For this review, take the finished solid that the model builds, in its own axes (mm). Coordinates: 2 decimals unless noted, no trailing zeros. Write each loop counter-clockwise with the first axis right and the second up, starting at its lowest first coordinate (ties: lowest second). Pieces come first, ordered by that corner, then holes. Notation, with made-up numbers: (36, 23.5) - (78, 23.5) arc R33 ccw to (78, 62.5) - close; hole circle Ø7 at (4.5, 57). An arc over 180 degrees is marked (long way). Use one line per item in the form item = value. Start each with the question number.
1) We need section A-A (x = -55). Give the boundary of the cut face in (y, z).
2) We need section C-C (x = -145). Give the boundary of the cut face in (y, z).
3) For L1, parallel to Y at x = -15, z = 0.6; L2, parallel to X at y = 55, z = 0.85; L3, parallel to Y at x = -145, z = 1, list the stretches that pass through material, from the lowest coordinate up. Write a range as from..to.
4) We need section B-B (y = 15). Give the boundary of the cut face in (x, z), plus the area to 3 significant figures.
5) Insertion check: P1, Ø0.8, axis at y = 19.5, z = 1.5, coming from the -X side; P2, Ø5.5, axis at x = -15, y = 10, coming from the +Z side. Each pin has a flat end and moves straight along its axis. Give the tip position at first contact, or say it passes through.
6) We need section D-D (y = 23). Give the boundary of the cut face in (x, z), plus the area to 3 significant figures.
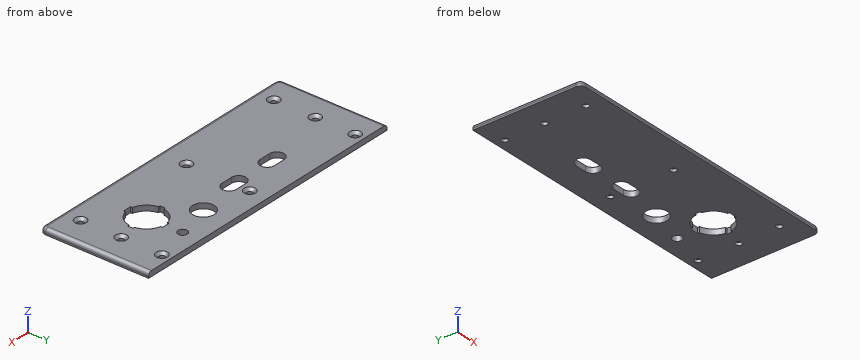
```python
from build123d import *

# Parameters (mm, degrees)
SKETCH11_W                                     = 160
SKETCH11_H                                     = 60
SKETCH11_R                                     = 2.55
SKETCH11_R_2                                   = 6
BOSS_EXTRUDE1_DEPTH                            = 3
FILLET1_R                                      = 2
FILLET3_R                                      = 3
CSK_FOR_M3_FLAT_HEAD_MACHINE_SCREW1_AT_2_COUNT = 2
CSK_FOR_M3_FLAT_HEAD_MACHINE_SCREW1_AT_2_PITCH = 22.022525482
CSK_FOR_M3_FLAT_HEAD_MACHINE_SCREW1_AT_3_COUNT = 2
CSK_FOR_M3_FLAT_HEAD_MACHINE_SCREW1_AT_3_PITCH = 45
CSK_FOR_M3_FLAT_HEAD_MACHINE_SCREW1_AT_4_COUNT = 2
CSK_FOR_M3_FLAT_HEAD_MACHINE_SCREW1_AT_4_PITCH = 137.490256535
CSK_FOR_M3_FLAT_HEAD_MACHINE_SCREW1_AT_5_COUNT = 2
CSK_FOR_M3_FLAT_HEAD_MACHINE_SCREW1_AT_5_PITCH = 131.892243209
CSK_FOR_M3_FLAT_HEAD_MACHINE_SCREW1_AT_6_COUNT = 2
CSK_FOR_M3_FLAT_HEAD_MACHINE_SCREW1_AT_6_PITCH = 130.000219213
CSK_FOR_M3_FLAT_HEAD_MACHINE_SCREW1_AT_7_COUNT = 2
CSK_FOR_M3_FLAT_HEAD_MACHINE_SCREW1_AT_7_PITCH = 65.174148425
CSK_FOR_M3_FLAT_HEAD_MACHINE_SCREW1_AT_8_COUNT = 2
CSK_FOR_M3_FLAT_HEAD_MACHINE_SCREW1_AT_8_PITCH = 76.196837301


with BuildPart() as part:
    # Sketch11 → Boss-Extrude1 (new body)
    with BuildSketch(Plane.XY):
        with Locations((-80, 30)):
            Rectangle(SKETCH11_W, SKETCH11_H)
        with Locations((-35, 50)):
            Circle(SKETCH11_R, mode=Mode.SUBTRACT)
        with Locations((-55, 45)):
            Circle(SKETCH11_R_2, mode=Mode.SUBTRACT)
        with BuildLine():
            Line((-44.886859967, 31.5), (-45.897247359, 31.5))
            Line((-45.897247359, 31.5), (-45.897247359, 28.5))
            Line((-45.897247359, 28.5), (-44.886859967, 28.5))
            ThreePointArc((-44.886859967, 28.5), (-42.370691635, 23.241826814), (-37.35, 20.280046296))
            Line((-37.35, 20.280046296), (-37.35, 19.253954216))
            Line((-37.35, 19.253954216), (-32.65, 19.253954216))
            Line((-32.65, 19.253954216), (-32.65, 20.280046296))
            ThreePointArc((-32.65, 20.280046296), (-27.629308365, 23.241826814), (-25.113140033, 28.5))
            Line((-25.113140033, 28.5), (-24.102752641, 28.5))
            Line((-24.102752641, 28.5), (-24.102752641, 31.5))
            Line((-24.102752641, 31.5), (-25.113140033, 31.5))
            ThreePointArc((-25.113140033, 31.5), (-27.629308365, 36.758173186), (-32.65, 39.719953704))
            Line((-32.65, 39.719953704), (-32.65, 40.746045784))
            Line((-32.65, 40.746045784), (-37.35, 40.746045784))
            Line((-37.35, 40.746045784), (-37.35, 39.719953704))
            ThreePointArc((-37.35, 39.719953704), (-42.370691635, 36.758173186), (-44.886859967, 31.5))
        make_face(mode=Mode.SUBTRACT)
        with BuildLine():
            Line((-83.627304882, 44.930328357), (-77.227304882, 44.930328357))
            ThreePointArc((-77.227304882, 44.930328357), (-73.227304882, 40.930328357), (-77.227304882, 36.930328357))
            Line((-77.227304882, 36.930328357), (-83.627304882, 36.930328357))
            ThreePointArc((-83.627304882, 36.930328357), (-87.627304882, 40.930328357), (-83.627304882, 44.930328357))
        make_face(mode=Mode.SUBTRACT)
        with BuildLine():
            Line((-109.252753418, 44.9), (-102.852753418, 44.9))
            ThreePointArc((-102.852753418, 44.9), (-98.852753418, 40.9), (-102.852753418, 36.9))
            Line((-102.852753418, 36.9), (-109.252753418, 36.9))
            ThreePointArc((-109.252753418, 36.9), (-113.252753418, 40.9), (-109.252753418, 44.9))
        make_face(mode=Mode.SUBTRACT)
    extrude(amount=BOSS_EXTRUDE1_DEPTH)

    # Fillet1
    fillet1_edges = [part.edges().sort_by_distance(p)[0] for p in [
        (-160, 30, 3),
        (-80, 0, 3),
        (0, 30, 3),
    ]]
    fillet(fillet1_edges, radius=FILLET1_R)

    # Fillet3
    # the kernel refuses this fillet: 3 mm, written as the material it takes off along each edge
    with BuildSketch(Plane(origin=(-3, 3, 3), x_dir=(0, -1, 0), z_dir=(-1, 0, 0))) as fillet3_piece_1:
        with BuildLine():
            CenterArc((1, -2), 2, 0, 90)
            Line((3, -2), (3, 0))
            Line((3, 0), (1, 0))
        make_face()
    revolve(axis=Axis((-3, 3, 3), (0, 0, 1)), revolution_arc=90, mode=Mode.SUBTRACT)
    with BuildSketch(Plane(origin=(-157, 3, 3), x_dir=(-1, 0, 0), z_dir=(0, 1, 0))) as fillet3_piece_2:
        with BuildLine():
            CenterArc((1, -2), 2, 0, 90)
            Line((3, -2), (3, 0))
            Line((3, 0), (1, 0))
        make_face()
    revolve(axis=Axis((-157, 3, 3), (0, 0, 1)), revolution_arc=90, mode=Mode.SUBTRACT)
    with BuildSketch(Plane(origin=(0, 0, -7.5), x_dir=(-1, 0, 0), z_dir=(0, 0, 1))) as fillet3_piece_3:
        with BuildLine():
            CenterArc((FILLET3_R, -FILLET3_R), FILLET3_R, 90, 90)
            Line((0, -FILLET3_R), (0, 0))
            Line((0, 0), (FILLET3_R, 0))
        make_face()
    extrude(amount=10.5, mode=Mode.SUBTRACT)
    with BuildSketch(Plane(origin=(-160, 0, -7.5), x_dir=(1, 0, 0), z_dir=(0, 0, 1))) as fillet3_piece_4:
        with BuildLine():
            CenterArc((FILLET3_R, FILLET3_R), FILLET3_R, 180, 90)
            Line((0, FILLET3_R), (0, 0))
            Line((0, 0), (FILLET3_R, 0))
        make_face()
    extrude(amount=10.5, mode=Mode.SUBTRACT)

    # Sketch13 → CSK for M3 Flat Head Machine Screw1 (revolve, cut)
    with BuildSketch(Plane(origin=(-145, 54.761262741, 3), x_dir=(0, -1, 0), z_dir=(1, 0, 0))):
        Polygon((0, 0), (0, 3), (1.7, 3), (1.7, 1.45), (3.15, 0), align=None)
    csk_for_m3_flat_head_machine_screw1 = revolve(axis=Axis((-145, 54.761262741, 9.35), (0, 0, -1)), mode=Mode.SUBTRACT)

    # CSK for M3 Flat Head Machine Screw1 at 2: CSK for M3 Flat Head Machine Screw1 ×2
    with Locations(*[(0, -i * CSK_FOR_M3_FLAT_HEAD_MACHINE_SCREW1_AT_2_PITCH, 0) for i in range(1, CSK_FOR_M3_FLAT_HEAD_MACHINE_SCREW1_AT_2_COUNT)]):
        add(csk_for_m3_flat_head_machine_screw1, mode=Mode.SUBTRACT)

    # CSK for M3 Flat Head Machine Screw1 at 3: CSK for M3 Flat Head Machine Screw1 ×2
    with Locations(*[(0, -i * CSK_FOR_M3_FLAT_HEAD_MACHINE_SCREW1_AT_3_PITCH, 0) for i in range(1, CSK_FOR_M3_FLAT_HEAD_MACHINE_SCREW1_AT_3_COUNT)]):
        add(csk_for_m3_flat_head_machine_screw1, mode=Mode.SUBTRACT)

    # CSK for M3 Flat Head Machine Screw1 at 4: CSK for M3 Flat Head Machine Screw1 ×2
    with Locations(*[Vector(0.9455215465875816, -0.3255595259528246, 0) * (i * CSK_FOR_M3_FLAT_HEAD_MACHINE_SCREW1_AT_4_PITCH) for i in range(1, CSK_FOR_M3_FLAT_HEAD_MACHINE_SCREW1_AT_4_COUNT)]):
        add(csk_for_m3_flat_head_machine_screw1, mode=Mode.SUBTRACT)

    # CSK for M3 Flat Head Machine Screw1 at 5: CSK for M3 Flat Head Machine Screw1 ×2
    with Locations(*[Vector(0.9856531122424032, -0.16878371463759412, 0) * (i * CSK_FOR_M3_FLAT_HEAD_MACHINE_SCREW1_AT_5_PITCH) for i in range(1, CSK_FOR_M3_FLAT_HEAD_MACHINE_SCREW1_AT_5_COUNT)]):
        add(csk_for_m3_flat_head_machine_screw1, mode=Mode.SUBTRACT)

    # CSK for M3 Flat Head Machine Screw1 at 6: CSK for M3 Flat Head Machine Screw1 ×2
    with Locations(*[Vector(0.9999983137474917, 0.0018364373589019598, 0) * (i * CSK_FOR_M3_FLAT_HEAD_MACHINE_SCREW1_AT_6_PITCH) for i in range(1, CSK_FOR_M3_FLAT_HEAD_MACHINE_SCREW1_AT_6_COUNT)]):
        add(csk_for_m3_flat_head_machine_screw1, mode=Mode.SUBTRACT)

    # CSK for M3 Flat Head Machine Screw1 at 7: CSK for M3 Flat Head Machine Screw1 ×2
    with Locations(*[Vector(0.9973279524332378, -0.0730544680038502, 0) * (i * CSK_FOR_M3_FLAT_HEAD_MACHINE_SCREW1_AT_7_PITCH) for i in range(1, CSK_FOR_M3_FLAT_HEAD_MACHINE_SCREW1_AT_7_COUNT)]):
        add(csk_for_m3_flat_head_machine_screw1, mode=Mode.SUBTRACT)

    # CSK for M3 Flat Head Machine Screw1 at 8: CSK for M3 Flat Head Machine Screw1 ×2
    with Locations(*[Vector(0.8530537788971958, -0.5218230066882967, 0) * (i * CSK_FOR_M3_FLAT_HEAD_MACHINE_SCREW1_AT_8_PITCH) for i in range(1, CSK_FOR_M3_FLAT_HEAD_MACHINE_SCREW1_AT_8_COUNT)]):
        add(csk_for_m3_flat_head_machine_screw1, mode=Mode.SUBTRACT)


solid = part.part
```
Determined:
q1.outline = (0, 0) - (39, 0) - (39, 3) - (2, 3) arc R2 ccw to (0, 1) - close; (51, 0) - (60, 0) - (60, 3) - (51, 3) - close
q2.outline = (0, 0) - (8.06, 0) - (8.06, 1.55) - (6.61, 3) - (2, 3) arc R2 ccw to (0, 1) - close; (11.46, 0) - (31.04, 0) - (31.04, 1.55) - (29.59, 3) - (12.91, 3) - (11.46, 1.55) - close; (34.44, 0) - (53.06, 0) - (53.06, 1.55) - (51.61, 3) - (35.89, 3) - (34.44, 1.55) - close; (56.46, 0) - (60, 0) - (60, 3) - (57.91, 3) - (56.46, 1.55) - close
q3.L1 = 0..8.3, 11.7..30.8, 34.2..53.3, 56.7..60
q3.L2 = -160..-146.68, -143.32..-16.7, -13.3..0
q3.L3 = 0..8.06, 11.46..31.04, 34.44..53.06, 56.46..60
q4.outline = (-160, 0) - (-81.7, 0) - (-81.7, 1.55) - (-83.15, 3) - (-158, 3) arc R2 ccw to (-160, 1) - close; (-78.3, 0) - (0, 0) - (0, 1) arc R2 ccw to (-2, 3) - (-76.85, 3) - (-78.3, 1.55) - close
q4.area = 466 mm²
q5.P1 = -160
q5.P2 = 2.6
q6.outline = (-160, 0) - (-42.14, 0) - (-42.14, 3) - (-158, 3) arc R2 ccw to (-160, 1) - close; (-27.86, 0) - (0, 0) - (0, 1) arc R2 ccw to (-2, 3) - (-27.86, 3) - close
q6.area = 435 mm²
